The model under review builds one solid part; all positions refer to its coordinate system, in mm. A direction names the side the tool comes from. Coordinates: 2 decimals unless noted, no trailing zeros. Write each loop counter-clockwise with the first axis right and the second up, starting at its lowest first coordinate (ties: lowest second). Pieces come first, ordered by that corner, then holes. Notation, with made-up numbers: (54, 18) - (78, 18) arc R22 cw to (78, 49) - close; hole circle Ø4 at (74, 86.25). An arc over 180 degrees is marked (long way). Put each result on its own line as item: value. Start each with the question number.
Item 1: For pin 1 (6.5 mm diameter, centred on x = 4.5, z = -16.5, fed in from -Y); pin 2 (2.5 mm diameter, centred on x = 37, z = -20.5, fed in from +Y); pin 3 (1.4 mm diameter, centred on x = -12, y = -1, fed in from +Z), all flat-tipped, find the tip position at first contact; note any pin that passes through.
Item 2: Consider section B-B on z = 13. Give the boundary of the cut face in (x, y).
Item 3: Mouldability with a two-part tool opening along Z and no side actions: class faces 4 (the face through (-1, 7, -30.25)), 5 (the face through (37, 5, -18)), 6 (the face through (-1, -2, 4.4)), 7 (the face through (-1, -4.8, -7)) as pulls with the +Z half, pulls with the -Z half, needs draft (parallel to the pull), parting line crosses it, or undercut.
Item 4: Consider section A-A on y = 3.25. Give the boundary of the cut face in (x, z).
Item 5: Consider section C-C on x = -15.5. Give the boundary of the cut face in (y, z).
Item 6: Machinability: for faces 1 (the face through (-1, -2, -4.4)), 2 (the face through (37, 9, -13.15)), 3 (the face through (-35.25, 8, 0)), which of the approach directions +Z, -Z, +X, -X, +Y, -Y give a long, thin tool a straight path to every point of the face, cutting with its end or side? Answer none if there is none.
Item 7: Consider section D-D on y = -2.75. Give the boundary of the cut face in (x, z), then the cut area to 4 significant figures.
Item 8: To check wall thickness, follow L1, parallel to X at y = 4, z = -9; L2, parallel to Z at x = -11, y = 10; L3, parallel to Z at x = -30, y = -1. State the ranges of each line that lie inside material, in increasing order. Write a range as [from, to].
```python
from build123d import *

# Parameters (mm, degrees)
SKETCH1_W           = 76.5
SKETCH1_H           = 60.5
BOSS_EXTRUDE1_DEPTH = 14
SKETCH2_W           = 70.5
SKETCH2_H           = 54.5
CUT_EXTRUDE1_DEPTH  = 12
CUT_EXTRUDE2_REACH  = 85.446
SKETCH4_W           = 13
SKETCH4_H           = 9
SKETCH4_W_2         = 10.2
SKETCH5_W           = 76.5
SKETCH5_H           = 4.5
BOSS_EXTRUDE3_DEPTH = 4.8


with BuildPart() as part:
    # Sketch1 → Boss-Extrude1 (new body)
    with BuildSketch(Plane(origin=(0, 0, 0), x_dir=(1, 0, 0), z_dir=(0, 1, 0))):
        Rectangle(SKETCH1_W, SKETCH1_H)
    extrude(amount=BOSS_EXTRUDE1_DEPTH)

    # Sketch2 → Cut-Extrude1 (cut)
    with BuildSketch(Plane(origin=(0, 14, 0), x_dir=(1, 0, 0), z_dir=(0, 1, 0))):
        Rectangle(SKETCH2_W, SKETCH2_H)
    extrude(amount=-CUT_EXTRUDE1_DEPTH, mode=Mode.SUBTRACT)

    # Sketch4 → Cut-Extrude2 (cut, up to next)
    with BuildSketch(Plane(origin=(38.25, 0, 0), x_dir=(0, 0, -1), z_dir=(1, 0, 0)), mode=Mode.PRIVATE) as cut_extrude2_sk1:
        with Locations((-11.55, 9.5)):
            Rectangle(SKETCH4_W, SKETCH4_H)
    cut_extrude2_tool1 = extrude(cut_extrude2_sk1.sketch, amount=-CUT_EXTRUDE2_REACH, mode=Mode.PRIVATE) & part.part
    # Sketch4 → Cut-Extrude2 (cut, up to next)
    with BuildSketch(Plane(origin=(38.25, 0, 0), x_dir=(0, 0, -1), z_dir=(1, 0, 0)), mode=Mode.PRIVATE) as cut_extrude2_sk2:
        with Locations((18.25, 9.5)):
            Rectangle(SKETCH4_W_2, SKETCH4_H)
    cut_extrude2_tool2 = extrude(cut_extrude2_sk2.sketch, amount=-CUT_EXTRUDE2_REACH, mode=Mode.PRIVATE) & part.part
    add(cut_extrude2_tool1.solids().sort_by_distance((38.25, 9.5, 11.55))[0], mode=Mode.SUBTRACT)
    add(cut_extrude2_tool2.solids().sort_by_distance((38.25, 9.5, -18.25))[0], mode=Mode.SUBTRACT)

    # Sketch5 → Boss-Extrude3 (add)
    with BuildSketch(Plane.XZ):
        with Locations((0, 6.65)):
            Rectangle(SKETCH5_W, SKETCH5_H)
    boss_extrude3 = extrude(amount=BOSS_EXTRUDE3_DEPTH)

    # Mirror1: Boss-Extrude3 across plane
    add(boss_extrude3.mirror(Plane.XY))


solid = part.part
```
Report:
1. pin 1: y = 0
1. pin 2: y = 5
1. pin 3: z = 8.9
2. outline: (-38.25, 0) - (38.25, 0) - (38.25, 5) - (35.25, 5) - (35.25, 2) - (-35.25, 2) - (-35.25, 14) - (-38.25, 14) - close
3. face 4: pulls with the -Z half
3. face 5: undercut
3. face 6: undercut
3. face 7: needs draft
4. outline: (-38.25, -30.25) - (38.25, -30.25) - (38.25, 30.25) - (-38.25, 30.25) - close; hole (-35.25, -27.25) - (35.25, -27.25) - (35.25, 27.25) - (-35.25, 27.25) - close
5. outline: (-4.8, -8.9) - (0, -8.9) - (0, -30.25) - (14, -30.25) - (14, -27.25) - (2, -27.25) - (2, 27.25) - (14, 27.25) - (14, 30.25) - (0, 30.25) - (0, 8.9) - (-4.8, 8.9) - (-4.8, 4.4) - (0, 4.4) - (0, -4.4) - (-4.8, -4.4) - close
6. face 1: +X, -X, -Y
6. face 2: +X, +Y
6. face 3: +Y
7. outline: (-38.25, -8.9) - (38.25, -8.9) - (38.25, -4.4) - (-38.25, -4.4) - close; (-38.25, 4.4) - (38.25, 4.4) - (38.25, 8.9) - (-38.25, 8.9) - close
7. area: 688.5 mm²
8. L1: [-38.25, -35.25], [35.25, 38.25]
8. L2: [-30.25, -27.25], [27.25, 30.25]
8. L3: [-8.9, -4.4], [4.4, 8.9]
